from build123d import *

# Parameters (mm, degrees)
F1_DEPTH = 8
F3_DEPTH = 25
F4_R     = 3.733765
F5_DEPTH = 2.5


with BuildPart() as f1:
    # F0 (on Front) → F1 (new body)
    with BuildSketch(Plane.XZ):
        Polygon((16.5, 1.75), (14, 1.75), (-14, 1.75), (-16.5, 1.75), (-16.5, 0), (0, 0), (16.5, 0), align=None)
        with BuildLine():
            Line((14, 4.25), (14, 1.75))
            Line((14, 1.75), (16.5, 1.75))
            Line((16.5, 1.75), (16.5, 2.25))
            ThreePointArc((16.5, 2.25), (15.085786, 2.835786), (14.5, 4.25))
            Line((14.5, 4.25), (14, 4.25))
        make_face()
        with BuildLine():
            Line((-16.5, 1.75), (-14, 1.75))
            Line((-14, 1.75), (-14, 4.25))
            Line((-14, 4.25), (-14.5, 4.25))
            ThreePointArc((-14.5, 4.25), (-15.085786, 2.835786), (-16.5, 2.25))
            Line((-16.5, 2.25), (-16.5, 1.75))
        make_face()
        with BuildLine():
            Line((16.5, 2.25), (16.5, 1.75))
            Line((16.5, 1.75), (20, 1.75))
            Line((20, 1.75), (20, 4.25))
            Line((20, 4.25), (18.5, 4.25))
            ThreePointArc((18.5, 4.25), (17.914214, 2.835786), (16.5, 2.25))
        make_face()
        Polygon((20, 1.75), (16.5, 1.75), (16.5, 0), (0, 0), (-16.5, 0), (-16.5, 1.75), (-20, 1.75), (-20, -1.75), (20, -1.75), align=None)
        with BuildLine():
            Line((14, 6.75), (14, 4.25))
            Line((14, 4.25), (14.5, 4.25))
            ThreePointArc((14.5, 4.25), (16.5, 6.25), (18.5, 4.25))
            Line((18.5, 4.25), (20, 4.25))
            Line((20, 4.25), (20, 6.75))
            Line((20, 6.75), (14, 6.75))
        make_face()
        with BuildLine():
            Line((-20, 1.75), (-16.5, 1.75))
            Line((-16.5, 1.75), (-16.5, 2.25))
            ThreePointArc((-16.5, 2.25), (-17.914214, 2.835786), (-18.5, 4.25))
            Line((-18.5, 4.25), (-20, 4.25))
            Line((-20, 4.25), (-20, 1.75))
        make_face()
        with BuildLine():
            Line((-14.5, 4.25), (-14, 4.25))
            Line((-14, 4.25), (-14, 6.75))
            Line((-14, 6.75), (-20, 6.75))
            Line((-20, 6.75), (-20, 4.25))
            Line((-20, 4.25), (-18.5, 4.25))
            ThreePointArc((-18.5, 4.25), (-16.5, 6.25), (-14.5, 4.25))
        make_face()
    extrude(amount=F1_DEPTH)

    # F2 (on face) → F3 (cut)
    with BuildSketch(Plane.XY.offset(1.75)):
        with BuildLine():
            ThreePointArc((1.75, -4), (1.237437, -2.762563), (0, -2.25))
            ThreePointArc((0, -2.25), (-1.237437, -5.237437), (1.75, -4))
        make_face()
    extrude(amount=-F3_DEPTH, mode=Mode.SUBTRACT)

    # F4 (on face) → F5 (cut)
    with BuildSketch(Plane.XY.offset(1.75)):
        with Locations((0, -4)):
            Circle(F4_R)
    extrude(amount=-F5_DEPTH, mode=Mode.SUBTRACT)


solid = f1.part
Source: CAD feature listing. Evaluate the final solid. Frame: model axes, mm. A direction names the side the tool comes from. Round coordinates to 2 decimals unless told otherwise and drop trailing zeros. Loops run counter-clockwise (first coordinate to the right, second up) from the corner with the lowest first, then second, coordinate; pieces in that order, holes last. Notation, with made-up numbers: M 64,-32 L 108,-32 A27 cw 108,2 Z; hole C 2,26.25 d3. An arc over 180 degrees is marked long. Return JSON: item names as keys, results as strings. Group by question number.
1. Section query D-D on z = 3. Output: boundary loops of the cut face in (x, y).
2. Section query C-C on y = -1. Output: boundary loops of the cut face in (x, z), and give its area (3 significant figures).
3. Material intervals for line 1 along Y through (x, z) = (0, -0.05); line 2 along X through (y, z) = (-3.75, 0.75); line 3 along Y through (x, z) = (0, -1.1), sorted ascending. Write a range as from..to.
4. Section query A-A on y = -3. Output: boundary loops of the cut face in (x, z).
5. Section query B-B on z = -0.25. Output: boundary loops of the cut face in (x, y), and give its area (3 significant figures).
6. Pin query (flat end, axial travel): pin 1 (5 mm diameter, centred on x = 8.5, z = 5.5, fed in from +Y); pin 2 (3.5 mm diameter, centred on x = -0.5, y = -4, fed in from +Z). Return the tip coordinate at first contact, or that it passes through.
7. Reachability of faces 1 (the face through (-0.809, -7.645, 0.518)), 2 (the face through (-20, -4, 3)), 3 (the face through (3, -1, 1.75)) from +Z, -Z, +X, -X, +Y, -Y: full face, straight path, thin tool, end or side. Return the list, or none.
Checks:
{
 "1": {"outline": "M -20,-8 L -18.06,-8 L -18.06,0 L -20,0 Z; M -14.94,-8 L -14,-8 L -14,0 L -14.94,0 Z; M 14,-8 L 14.94,-8 L 14.94,0 L 14,0 Z; M 18.06,-8 L 20,-8 L 20,0 L 18.06,0 Z"},
 "2": {"outline": "M -20,-1.75 L 20,-1.75 L 20,6.75 L 14,6.75 L 14,1.75 L 2.22,1.75 L 2.22,-0.75 L -2.22,-0.75 L -2.22,1.75 L -14,1.75 L -14,6.75 L -20,6.75 Z; hole M -18.5,4.25 A2 ccw -16.5,2.25 A2 ccw -14.5,4.25 A2 ccw Z; hole M 14.5,4.25 A2 ccw 16.5,2.25 A2 ccw 18.5,4.25 A2 ccw Z", "area": "164 mm²"},
 "3": {"line 1": "y = -8..-7.73, -0.27..0", "line 2": "x = -20..-3.73, 3.73..20", "line 3": "y = -8..-5.75, -2.25..0"},
 "4": {"outline": "M -20,-1.75 L -1.44,-1.75 L -1.44,-0.75 L -3.6,-0.75 L -3.6,1.75 L -14,1.75 L -14,6.75 L -20,6.75 Z; M 1.44,-1.75 L 20,-1.75 L 20,6.75 L 14,6.75 L 14,1.75 L 3.6,1.75 L 3.6,-0.75 L 1.44,-0.75 Z; hole M -18.5,4.25 A2 ccw -16.5,2.25 A2 ccw -14.5,4.25 A2 ccw Z; hole M 14.5,4.25 A2 ccw 16.5,2.25 A2 ccw 18.5,4.25 A2 ccw Z"},
 "5": {"outline": "M -20,-8 L 20,-8 L 20,0 L -20,0 Z; hole C 0,-4 d7.47", "area": "276 mm²"},
 "6": {"pin 1": "passes through", "pin 2": "stops at z = -0.75"},
 "7": {"face 1": "+Z", "face 2": "+Z, -Z, -X, +Y, -Y", "face 3": "+Z, +Y, -Y"}
}
